Can you work these out from the model? Positions are in its coordinate system, mm. Face numbers are marked on the shaded views. A direction names the side the tool comes from. Give positions to 0.01 mm unless a question says otherwise; leave off trailing zeros. Loops run counter-clockwise (first coordinate to the right, second up) from the corner with the lowest first, then second, coordinate; pieces in that order, holes last. Notation, with made-up numbers: (67.25, 6.25) - (78.25, 6.25) arc R23 ccw to (78.25, 15.25) - close; hole circle Ø10 at (71, 45.5). An arc over 180 degrees is marked (long way). Answer as a JSON object with one key per item and string values. Group by question number.
Item 1: Suppose I cut it at A-A on z = 75.25. Write out the boundary of the cut face in (x, y) (3 decimals).
Item 2: Which directions (+Z, -Z, +X, -X, +Y, -Y) give clear straight access to the entire face, cutting with the end or side of a thin tool? Please do the marked faces 1 and 2.
Item 3: Will these pins go through, and if not, where does the flat tip stop? pin 1 (1.6 mm diameter, centred on x = -12.15, y = 268.29, fed in from -Z); pin 2 (2 mm diameter, centred on y = 180.5, z = 73, fed in from -X); pin 3 (4.5 mm diameter, centred on y = 219, z = 76.5, fed in from +X).
Item 4: Suppose I cut it at C-C on x = -2.5. Write out the boundary of the cut face in (y, z) (3 decimals), and give its area (3 significant figures).
Item 5: Please list where these lines run through material, in increasing order: L1, parallel to X at y = 214, z = 80.25; L2, parallel to X at y = 201.5, z = 75.25; L3, parallel to Z at x = -12.75, y = 213.
from build123d import *

# Parameters (mm, degrees)
BOSS_EXTRUDE1_DEPTH = 431.8
FILLET2_R           = 12.7
SKETCH2_R           = 2.032
CUT_EXTRUDE1_DEPTH  = 436.166892099
SCALE1_SCALE        = 0.25


with BuildPart() as part:
    # Sketch1 → Boss-Extrude1 (new body)
    with BuildSketch(Plane(origin=(0, 0, 0), x_dir=(1, 0, 0), z_dir=(0, 1, 0))):
        with BuildLine():
            Line((12.446, -95.666893232), (12.446, -83.267976842))
            ThreePointArc((12.446, -83.267976842), (12.103082443, -66.082532596), (-4.162019583, -60.523437125))
            Line((-4.162019583, -60.523437125), (-20.574, -65.268050741))
            Line((-20.574, -65.268050741), (-20.574, -84.572180345))
            Line((-20.574, -84.572180345), (-20.574, -95.666893232))
            Line((-20.574, -95.666893232), (-39.624, -95.666893232))
            Line((-39.624, -95.666893232), (-39.624, -92.491893232))
            Line((-39.624, -92.491893232), (-26.924, -92.491893232))
            Line((-26.924, -92.491893232), (-26.924, -62.093050741))
            ThreePointArc((-26.924, -62.093050741), (-4.064, -55.764211531), (18.796, -62.093050741))
            Line((18.796, -62.093050741), (18.796, -92.491893232))
            Line((18.796, -92.491893232), (31.496, -92.491893232))
            Line((31.496, -92.491893232), (31.496, -95.666893232))
            Line((31.496, -95.666893232), (12.446, -95.666893232))
        make_face()
    extrude(amount=BOSS_EXTRUDE1_DEPTH)

    # Fillet2
    fillet2_edges = [part.edges().sort_by_distance(p)[0] for p in [
        (-26.924, 215.9, 62.093050741),
        (18.796, 215.9, 62.093050741),
    ]]
    fillet(fillet2_edges, radius=FILLET2_R)

    # Sketch2 → Cut-Extrude1 (cut, through all)
    with BuildSketch(Plane(origin=(0, 0, 92.491893232), x_dir=(-1, 0, 0), z_dir=(0, 0, -1))):
        with Locations((-25.146, 425.45)):
            Circle(SKETCH2_R)
        with Locations((-25.146, 6.35)):
            Circle(SKETCH2_R)
        with Locations((33.274, 425.45)):
            Circle(SKETCH2_R)
        with Locations((33.274, 6.35)):
            Circle(SKETCH2_R)
    extrude(amount=-CUT_EXTRUDE1_DEPTH, mode=Mode.SUBTRACT)


with BuildPart() as part_1:
    # Scale1: scaled about (-5.110319003, 215.9, 75.736877767)
    add(part.part.scale(SCALE1_SCALE).moved(Location((-3.832739252, 161.925, 56.802658325))))


solid = part_1.part
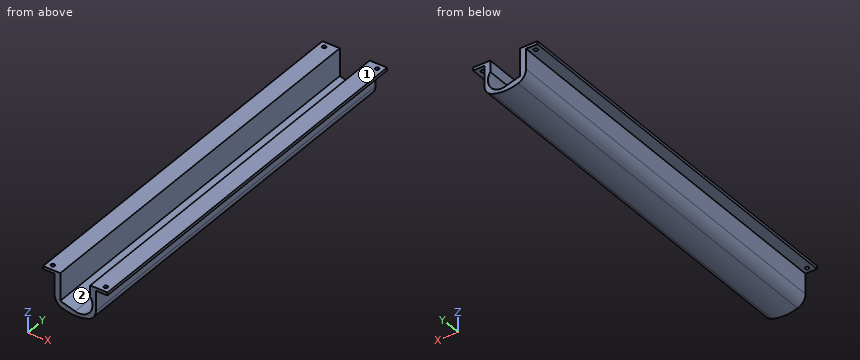
Worked out:
{
 "1": {"outline": "(-10.564, 161.925) - (-8.976, 161.925) - (-8.976, 269.875) - (-10.564, 269.875) - close; (-0.097, 161.925) - (0.866, 161.925) - (0.866, 269.875) - (-0.097, 269.875) - close"},
 "2": {"face 1": "+Z, +X, -X, +Y, -Y", "face 2": "+Z, +Y, -Y"},
 "3": {"pin 1": "stops at z = 79.93", "pin 2": "stops at x = -10.55", "pin 3": "stops at x = 0.87"},
 "4": {"outline": "(161.925, 70.995) - (269.875, 70.995) - (269.875, 72.031) - (161.925, 72.031) - close", "area": "112 mm2"},
 "5": {"L1": "x = -13.74 to -8.98, -0.72 to 4.04", "L2": "x = -10.56 to -8.98, -0.1 to 0.87", "L3": "z = 79.93 to 80.72"}
}
